from build123d import *

# Parameters (mm, degrees)
EXTRUDE_1_DEPTH     = 2.4
SKETCH_2_R          = 1.5
CUT_EXTRUDE_1_DEPTH = 5.510358448
CHAMFER_1_SIZE      = 0.3


with BuildPart() as part:
    # Эскиз1 → Вытянуть1 (new body)
    with BuildSketch(Plane(origin=(0, 0, 0), x_dir=(1, 0, 0), z_dir=(0, 1, 0))):
        Polygon((-1.443375673, 2.5), (1.443375673, 2.5), (2.886751346, 0), (1.443375673, -2.5), (-1.443375673, -2.5), (-2.886751346, 0), align=None)
    extrude(amount=-EXTRUDE_1_DEPTH)

    # Эскиз2 → Вырез-Вытянуть1 (cut, through all)
    with BuildSketch(Plane(origin=(0, 0, 0), x_dir=(-1, 0, 0), z_dir=(0, 1, 0))):
        with Locations(Location((0, 0, 0), (0, 0, 90))):
            Circle(SKETCH_2_R)
    extrude(amount=-CUT_EXTRUDE_1_DEPTH, mode=Mode.SUBTRACT)

    # Фаска1
    chamfer_1_edges = [part.edges().sort_by_distance(p)[0] for p in [
        (0, -2.4, -1.5),
        (0, 0, -1.5),
    ]]
    chamfer(chamfer_1_edges, length=CHAMFER_1_SIZE)

    # Эскиз3 → Вырез-Повернуть1 (revolve, cut)
    with BuildSketch(Plane.XY, mode=Mode.PRIVATE) as cut_revolve_1_sk:
        Polygon((-2.886751346, 0), (-2.486751346, 0), (-2.886751346, -0.4), align=None)
        Polygon((-2.886751346, -2), (-2.886751346, -2.4), (-2.486751346, -2.4), align=None)
    revolve(cut_revolve_1_sk.sketch.rotate(Axis((0, -0.3, 0), (0, -1, 0)), 120.000000241), axis=Axis((0, -0.3, 0), (0, -1, 0)), mode=Mode.SUBTRACT)


solid = part.part
Could you check a few things on this model? Use its own coordinates, in mm. Give positions to 0.01 mm unless a question says otherwise; leave off trailing zeros. Order: outer loops, then holes, each group sorted by start corner. A loop starts at its lowest first (then second) coordinate and runs counter-clockwise, first axis right, second up.
1. I need wall thicknesses on L1, parallel to X at y = -0.75, z = 1.25; L2, parallel to Z at x = 0.9, y = -1.5; L3, parallel to X at y = -0.7, z = -0.6. Which ranges of each line are inside material? Lowest first, please.
2. Suppose I cut it at B-B (y = -0.65). List the corners of the cut face in (x, z) for me, plus the area to 3 significant figures.
3. We'd pull the mould along Z, two halves only. Please class faces 1 (the flat face through (-2.175, -1.183, -1.233)), 2 (the flat face through (-2, -2.4, -1)), 3 (the cylindrical face through (0.45, -1.19, 1.43)): pulls with the +Z half, pulls with the -Z half, needs draft (parallel to the pull), parting line crosses it, or undercut.
Solved:
1. L1: x = -2.17 to -0.83, 0.83 to 2.17
1. L2: z = -2.5 to -1.2, 1.2 to 2.5
1. L3: x = -2.54 to -1.37, 1.37 to 2.54
2. outline: (-2.89, 0) - (-1.44, -2.5) - (1.44, -2.5) - (2.89, 0) - (1.44, 2.5) - (-1.44, 2.5) - close; hole circle Ø3 at (0, 0)
2. area: 14.6 mm2
3. face 1: pulls with the -Z half
3. face 2: needs draft
3. face 3: undercut
